from build123d import *

# Parameters (mm, degrees)
SKETCH1_R           = 10
BOSS_EXTRUDE1_DEPTH = 45
SKETCH2_R           = 14
BOSS_EXTRUDE2_DEPTH = 2
SKETCH3_R           = 14
BOSS_EXTRUDE3_DEPTH = 15


with BuildPart() as part:
    # Sketch1 → Boss-Extrude1 (new body)
    with BuildSketch(Plane(origin=(0, 0, 0), x_dir=(1, 0, 0), z_dir=(0, 1, 0))):
        Circle(SKETCH1_R)
    extrude(amount=BOSS_EXTRUDE1_DEPTH)

    # Sketch2 → Boss-Extrude2 (add)
    with BuildSketch(Plane(origin=(0, 45, 0), x_dir=(1, 0, 0), z_dir=(0, 1, 0))):
        Circle(SKETCH2_R)
    extrude(amount=BOSS_EXTRUDE2_DEPTH)

    # Sketch3 → Boss-Extrude3 (add)
    with BuildSketch(Plane(origin=(0, 47, 0), x_dir=(1, 0, 0), z_dir=(0, 1, 0))):
        Circle(SKETCH3_R)
        Polygon((11.542222646, -0.332309673), (6.058899942, 9.829703191), (-5.483322704, 10.162012864), (-11.542222646, 0.332309673), (-6.058899942, -9.829703191), (5.483322704, -10.162012864), align=None, mode=Mode.SUBTRACT)
    extrude(amount=BOSS_EXTRUDE3_DEPTH)


solid = part.part
Part model, mm, in its own coordinate system. A direction names the side the tool comes from. Coordinates: 2 decimals unless noted, no trailing zeros. Loops run counter-clockwise (first coordinate to the right, second up) from the corner with the lowest first, then second, coordinate; pieces in that order, holes last. Notation, with made-up numbers: (63, 68.25) -> (113, 68.25) arc R29 ccw to (113, 93.25) -> close; hole circle Ø5 at (88.25, 48). An arc over 180 degrees is marked (long way). Use a Markdown table: item, result. Add a question column.
Item 1: Band-saw the part on B-B on y = 14. Write the cut outline in (x, z), plus the area to 3 significant figures.
Item 2: Pull direction X, two halves, no side cores. Call faces 4 (the cylindrical face through (12.932, 53.381, 5.362)), 5 (the flat face through (0, 47, 0)), 6 (the flat face through (2, 62, -10.4)): +X half, -X half, draft (parallel to the pull), parting line (faces both ways), or undercut.
Item 3: Flat gauge pins, fed straight in: P1, Ø12, axis at x = 8, y = 34, coming from the +Z side; P2, Ø6, axis at x = 10.5, y = 33.5, coming from the -Z side; P3, Ø12, axis at x = -4, z = -3, coming from the +Y side; P4, Ø3, axis at x = 4, y = 39, coming from the +Z side. Where does each tip first touch, or does it go through?
Item 4: Which spindle directions (+Z, -Z, +X, -X, +Y, -Y) get a long thin tool onto all of the face, cutting with end or side? Do faces 1 (the flat face through (8.47, 54.4, 5.32)), 2 (the flat face through (-3, 45, -10)), 3 (the flat face through (0, 0, 0)). Say none if no direction does.
Item 5: Band-saw the part on A-A on z = -8.25. Write the cut outline in (x, y).
Item 6: Band-saw the part on C-C on x = 0. Write the cut outline in (y, z).
Item 7: Probe probe 1 along Z at (x, y) = (-0.5, 23); probe 2 along X at (y, z) = (58, 9.25); probe 3 along Y at (x, z) = (3, -8.75). List the from-to ranges inside material, lowest first.
Geometry says:
| question | item | result |
|---|---|---|
| 1 | outline | circle Ø20 at (0, 0) |
| 1 | area | 314 mm² |
| 2 | face 4 | parting line |
| 2 | face 5 | undercut |
| 2 | face 6 | draft |
| 3 | P1 | z = 9.8 |
| 3 | P2 | z = -6.61 |
| 3 | P3 | y = 62 |
| 3 | P4 | z = 9.68 |
| 4 | face 1 | +Y |
| 4 | face 2 | -Y |
| 4 | face 3 | +Z, -Z, +X, -X, -Y |
| 5 | outline | (-11.31, 45) -> (-5.65, 45) -> (-5.65, 0) -> (5.65, 0) -> (5.65, 45) -> (11.31, 45) -> (11.31, 62) -> (6.91, 62) -> (6.91, 47) -> (-6.66, 47) -> (-6.66, 62) -> (-11.31, 62) -> close |
| 6 | outline | (0, -10) -> (45, -10) -> (45, -14) -> (62, -14) -> (62, -10) -> (47, -10) -> (47, 10) -> (62, 10) -> (62, 14) -> (45, 14) -> (45, 10) -> (0, 10) -> close |
| 7 | probe 1 | -9.99 to 9.99 |
| 7 | probe 2 | -10.51 to -6.37, 6.05 to 10.51 |
| 7 | probe 3 | 0 to 47 |
